Read the model definition and answer for the solid it produces. Units are mm, in the model's axes. A direction names the side the tool comes from. Coordinates: 2 decimals unless noted, no trailing zeros. Write each loop counter-clockwise with the first axis right and the second up, starting at its lowest first coordinate (ties: lowest second). Pieces come first, ordered by that corner, then holes. Notation, with made-up numbers: (-15, 53.5) -> (14, 53.5) arc R11 cw to (14, 72.5) -> close; hole circle Ø4 at (-14, 17.25). An arc over 180 degrees is marked (long way). Use CSV: the item, a comma, the result in double quotes.
from build123d import *

# Parameters (mm, degrees)
SKETCH1_R               = 2
BOSS_EXTRUDE1_DEPTH     = 20
CHAMFER1_SIZE           = 0.5
SKETCH2_R               = 1
CUT_EXTRUDE1_DEPTH      = 3
CUT_EXTRUDE1_DEPTH_BACK = 3


with BuildPart() as part:
    # Sketch1 → Boss-Extrude1 (new body)
    with BuildSketch(Plane(origin=(0, 0, 0), x_dir=(0, 0, -1), z_dir=(1, 0, 0))):
        Circle(SKETCH1_R)
    extrude(amount=BOSS_EXTRUDE1_DEPTH)

    # Chamfer1
    chamfer1_edges = [part.edges().sort_by_distance(p)[0] for p in [
        (0, 0, 2),
    ]]
    chamfer(chamfer1_edges, length=CHAMFER1_SIZE)

    # Sketch2 → Cut-Extrude1 (cut, two sides)
    with BuildSketch(Plane(origin=(0, 0, 0), x_dir=(1, 0, 0), z_dir=(0, 1, 0))) as cut_extrude1_sk:
        with Locations((4, 0)):
            Circle(SKETCH2_R)
    extrude(amount=CUT_EXTRUDE1_DEPTH, mode=Mode.SUBTRACT)
    extrude(cut_extrude1_sk.sketch, amount=-CUT_EXTRUDE1_DEPTH_BACK, mode=Mode.SUBTRACT)

    # Sketch4 → Revolve1 (revolve)
    with BuildSketch(Plane.XY):
        with BuildLine():
            Line((20, 3.017004448), (20, 0))
            Line((20, 0), (22.6, 0))
            ThreePointArc((22.6, 0), (21.755214952, 1.900798256), (20, 3.017004448))
        make_face()
    revolve(axis=Axis((19, 0, 0), (1, 0, 0)))


solid = part.part
1. Find the intervals of material crossed by line 1 along X through (y, z) = (-0.75, 0); line 2 along Z through (x, y) = (4, -1.5); line 3 along X through (y, z) = (0, -0.25), in increasing order.
Solutions:
line 1,"x = 0 to 3, 5 to 22.42"
line 2,"z = -1.32 to -1, 1 to 1.32"
line 3,"x = 0 to 3.03, 4.97 to 22.56"
2. A cutting plane is placed at A-A (x = 4). Give the vertices of the cut face in (y, z).
Solutions:
outline,"(-1.73, -1) arc R2 ccw to (1.73, -1) -> close; (-1.73, 1) -> (1.73, 1) arc R2 ccw to start"
3. Each of these flat-tipped pins is pushed along its axis until it touches: pin 1 Ø3 at (x, z) = (7, 2) entering from -Y; pin 2 Ø3 at (x, z) = (16.5, 2) entering from +Y; pin 3 Ø2 at (x, z) = (9, 1) entering from +Y; pin 4 Ø1.6 at (x, z) = (4, 0) entering from -Y. Where does it stop, or does it pass through?
Solutions:
pin 1,"stops at y = -1.94"
pin 2,"stops at y = 1.94"
pin 3,"stops at y = 2"
pin 4,"passes through"
4. A tool of negligible diameter and unlimited length cuts with its end or side. For faces 1 (the flat face through (0, 0, 0)), 2 (the cylindrical face through (10.114, -0.766, -1.847)), from which of +Z, -Z, +X, -X, +Y, -Y can it reach the whole face along a straight path? Write none if from no direction.
Solutions:
face 1,"+Z, -Z, -X, +Y, -Y"
face 2,"-X"
